from build123d import *

# Parameters (mm, degrees)
F1_DEPTH = 12.7
F2_W     = 12.7
F2_H     = 50.8
F3_DEPTH = 25.4
F4_R     = 3.81
F5_DEPTH = 25.4


with BuildPart() as f1:
    # F0 (on Top) → F1 (new body)
    with BuildSketch(Plane.XY):
        Polygon((-12.7, 18.245806), (-12.7, -32.554194), (12.7, -32.554194), (12.7, 18.245806), (0, 40.242851), align=None)
    extrude(amount=F1_DEPTH)

    # F2 (on face) → F3 (join)
    with BuildSketch(Plane.XY.offset(12.7)):
        with Locations((0.299774, -1.667303)):
            Rectangle(F2_W, F2_H)
    extrude(amount=F3_DEPTH)

    # F4 (on face) → F5 (join)
    with BuildSketch(Plane.XY.offset(38.1)):
        with Locations((0.299774, 16.11553)):
            Circle(F4_R)
        with Locations((0.299774, 0.87553)):
            Circle(F4_R)
        with Locations((0.299774, -14.36447)):
            Circle(F4_R)
    extrude(amount=F5_DEPTH)


solid = f1.part
Here's how the part is built. I have some questions about the finished solid (model axes, mm). A direction names the side the tool comes from. Coordinates: 2 decimals unless noted, no trailing zeros. Order: outer loops, then holes, each group sorted by start corner. A loop starts at its lowest first (then second) coordinate and runs counter-clockwise, first axis right, second up.
Item 1: I need wall thicknesses on line 1 (Y direction, x = -1, z = 56); line 2 (Y direction, x = 0.25, z = 23); line 3 (X direction, y = -18.5, z = 35.5). Which ranges of each line are inside material? Lowest first, please.
Result sheet:
line 1: y = -17.95 to -10.78, -2.71 to 4.46, 12.53 to 19.7
line 2: y = -27.07 to 23.73
line 3: x = -6.05 to 6.65
Item 2: If we section it at C-C on z = 5: List the corners of the cut face in (x, y) for me.
Result sheet:
outline: (-12.7, -32.55) - (12.7, -32.55) - (12.7, 18.25) - (0, 40.24) - (-12.7, 18.25) - close
Item 3: If we mould it in two halves opening along Y, with no side actions, what happens to faces 1 (the face through (4, -1, 38.1)), 2 (the face through (-6.26, 29.4, 6.26)), 3 (the face through (-0.196, -10.587, 50.622)), 4 (the face through (-12.7, -7, 6))? For each: +Y half, -Y half, draft (parallel to the pull), parting line (faces both ways), or undercut.
Result sheet:
face 1: undercut
face 2: +Y half
face 3: undercut
face 4: draft
Item 4: For P1, Ø1.5, axis at y = -7.5, z = 33.5, coming from the -X side; P2, Ø8, axis at x = -5, z = 21.5, coming from the +Y side; P3, Ø4, axis at x = -3.5, z = 24.5, coming from the -Y side, each with a flat end and sliding along its axis, tell me the tip position at first contact or that it passes through.
Result sheet:
P1: stops at x = -6.05
P2: stops at y = 23.73
P3: stops at y = -27.07
Item 5: For faces 5 (the face through (0, -27.067, 25)), 6 (the face through (-6.05, -2, 25)), 7 (the face through (-0.526, -2.844, 50.622)), 8 (the face through (6.65, -2, 25)), 9 (the face through (0, 23.733, 25)), which set-ups out of +Z, -Z, +X, -X, +Y, -Y let a thin tool reach every point of the face, with its end or its side?
Result sheet:
face 5: +Z, +X, -X, -Y
face 6: +Z, -X, +Y, -Y
face 7: +Z
face 8: +Z, +X, +Y, -Y
face 9: +Z, +X, -X, +Y
Item 6: If we section it at B-B on x = 5.5: List the corners of the cut face in (y, z) for me.
Result sheet:
outline: (-32.55, 0) - (30.72, 0) - (30.72, 12.7) - (23.73, 12.7) - (23.73, 38.1) - (-27.07, 38.1) - (-27.07, 12.7) - (-32.55, 12.7) - close
Item 7: If we section it at D-D on z = 41.5: List the corners of the cut face in (x, y) for me, plus the area to 3 significant figures.
Result sheet:
outline: circle Ø7.62 at (0.3, -14.36); circle Ø7.62 at (0.3, 0.88); circle Ø7.62 at (0.3, 16.12)
area: 137 mm2
Item 8: If we section it at A-A on y = -25: List the corners of the cut face in (x, z) for me.
Result sheet:
outline: (-12.7, 0) - (12.7, 0) - (12.7, 12.7) - (6.65, 12.7) - (6.65, 38.1) - (-6.05, 38.1) - (-6.05, 12.7) - (-12.7, 12.7) - close
